Verification items for the finished model (mm, model axes). A direction names the side the tool comes from. Give positions to 0.01 mm unless a question says otherwise; leave off trailing zeros. Write each loop counter-clockwise with the first axis right and the second up, starting at its lowest first coordinate (ties: lowest second). Pieces come first, ordered by that corner, then holes. Notation, with made-up numbers: (-30, 24) - (8, 24) arc R19 ccw to (8, 45) - close; hole circle Ø3 at (6, -16.5). An arc over 180 degrees is marked (long way). Put each result on its own line as item: value.
from build123d import *

# Parameters (mm, degrees)
IZIM1_R                     = 1.5
IZIM1_R_2                   = 1.275
Y_KSEKLIK_EKSTR_ZYON1_DEPTH = 8
IZIM2_R                     = 4
KES_EKSTR_ZYON1_DEPTH       = 5
IZIM3_R                     = 3.5
KES_EKSTR_ZYON2_DEPTH       = 5
IZIM5_W                     = 11.833700998
IZIM5_H                     = 5.687133077
Y_KSEKLIK_EKSTR_ZYON2_DEPTH = 49
IZIM6_R                     = 1.5
KES_EKSTR_ZYON3_DEPTH       = 70
IZIM7_R                     = 7.94785764
KES_EKSTR_ZYON4_DEPTH       = 94.5
IZIM8_R                     = 2.303053837
IZIM8_R_2                   = 1.275
Y_KSEKLIK_EKSTR_ZYON3_DEPTH = 7
IZIM9_W                     = 9.184473095
IZIM9_H                     = 54.60219781
KES_EKSTR_ZYON5_DEPTH       = 49


with BuildPart() as part:
    # Çizim1 → Yükseklik-Ekstrüzyon1 (new body)
    with BuildSketch(Plane.XY):
        with BuildLine():
            Line((-26.942326891, 14.769848309), (-7.118223783, 14.769848309))
            ThreePointArc((-7.118223783, 14.769848309), (-3.582689877, 13.305382214), (-2.118223783, 9.769848309))
            Line((-2.118223783, 9.769848309), (-2.118223783, -8.006371062))
            ThreePointArc((-2.118223783, -8.006371062), (-3.582689877, -11.541904968), (-7.118223783, -13.006371062))
            Line((-7.118223783, -13.006371062), (-26.942326891, -13.006371062))
            ThreePointArc((-26.942326891, -13.006371062), (-30.477860797, -14.470837156), (-31.942326891, -18.006371062))
            Line((-31.942326891, -18.006371062), (-31.942326891, -21.470074229))
            ThreePointArc((-31.942326891, -21.470074229), (-31.6091093, -24.030019123), (-30.63166332, -26.419360282))
            Line((-30.63166332, -26.419360282), (-25.398075072, -35.607838889))
            ThreePointArc((-25.398075072, -35.607838889), (-21.734031643, -39.304154624), (-16.708738643, -40.658552836))
            Line((-16.708738643, -40.658552836), (16.824084861, -40.658552836))
            ThreePointArc((16.824084861, -40.658552836), (21.849377861, -39.304154624), (25.513421289, -35.607838889))
            Line((25.513421289, -35.607838889), (30.747009537, -26.419360282))
            ThreePointArc((30.747009537, -26.419360282), (31.724455518, -24.030019123), (32.057673109, -21.470074229))
            Line((32.057673109, -21.470074229), (32.057673109, -18.006371062))
            ThreePointArc((32.057673109, -18.006371062), (30.593207015, -14.470837156), (27.057673109, -13.006371062))
            Line((27.057673109, -13.006371062), (7.233570001, -13.006371062))
            ThreePointArc((7.233570001, -13.006371062), (3.698036095, -11.541904968), (2.233570001, -8.006371062))
            Line((2.233570001, -8.006371062), (2.233570001, 9.769848309))
            ThreePointArc((2.233570001, 9.769848309), (3.698036095, 13.305382214), (7.233570001, 14.769848309))
            Line((7.233570001, 14.769848309), (27.057673109, 14.769848309))
            ThreePointArc((27.057673109, 14.769848309), (30.593207015, 16.234314403), (32.057673109, 19.769848309))
            Line((32.057673109, 19.769848309), (32.057673109, 23.233551476))
            ThreePointArc((32.057673109, 23.233551476), (31.724455518, 25.793496369), (30.747009537, 28.182837528))
            Line((30.747009537, 28.182837528), (25.513421289, 37.371316135))
            ThreePointArc((25.513421289, 37.371316135), (21.849377861, 41.06763187), (16.824084861, 42.422030083))
            Line((16.824084861, 42.422030083), (-16.708738643, 42.422030083))
            ThreePointArc((-16.708738643, 42.422030083), (-21.734031643, 41.06763187), (-25.398075072, 37.371316135))
            Line((-25.398075072, 37.371316135), (-30.63166332, 28.182837528))
            ThreePointArc((-30.63166332, 28.182837528), (-31.6091093, 25.793496369), (-31.942326891, 23.233551476))
            Line((-31.942326891, 23.233551476), (-31.942326891, 19.769848309))
            ThreePointArc((-31.942326891, 19.769848309), (-30.477860797, 16.234314403), (-26.942326891, 14.769848309))
        make_face()
        with Locations((20.284256069, 32.422030083)):
            Circle(IZIM1_R, mode=Mode.SUBTRACT)
        with Locations((-20.168909852, 32.422030083)):
            Circle(IZIM1_R, mode=Mode.SUBTRACT)
        with Locations((-20.168909852, -30.658552836)):
            Circle(IZIM1_R, mode=Mode.SUBTRACT)
        with Locations((20.284256069, -30.658552836)):
            Circle(IZIM1_R, mode=Mode.SUBTRACT)
        with Locations((22.057673109, -21.118261377)):
            Circle(IZIM1_R_2, mode=Mode.SUBTRACT)
        with Locations((-21.942326891, -21.118261377)):
            Circle(IZIM1_R_2, mode=Mode.SUBTRACT)
        with Locations((22.057673109, 22.881738623)):
            Circle(IZIM1_R_2, mode=Mode.SUBTRACT)
        with Locations((-21.942326891, 22.881738623)):
            Circle(IZIM1_R_2, mode=Mode.SUBTRACT)
        with Locations((0.057673109, 32.422030083)):
            Circle(IZIM1_R, mode=Mode.SUBTRACT)
        with Locations(Location((0.057673109, -30.658552836, 0), (0, 0, 180))):
            Circle(IZIM1_R, mode=Mode.SUBTRACT)
    extrude(amount=Y_KSEKLIK_EKSTR_ZYON1_DEPTH)

    # Çizim2 → Kes-Ekstrüzyon1 (cut)
    with BuildSketch(Plane(origin=(0, 0, 0), x_dir=(-1, 0, 0), z_dir=(0, 0, -1))):
        with Locations((-22.057673109, 22.881738623)):
            Circle(IZIM2_R)
        with Locations((21.942326891, 22.881738623)):
            Circle(IZIM2_R)
        with Locations((-22.057673109, -21.118261377)):
            Circle(IZIM2_R)
        with Locations((21.942326891, -21.118261377)):
            Circle(IZIM2_R)
        with Locations((-0.057673109, 32.422030083)):
            Circle(IZIM2_R)
        with Locations((-0.057673109, -30.658552836)):
            Circle(IZIM2_R)
    extrude(amount=-KES_EKSTR_ZYON1_DEPTH, mode=Mode.SUBTRACT)

    # Çizim3 → Kes-Ekstrüzyon2 (cut)
    with BuildSketch(Plane.XY.offset(8)):
        with Locations((-20.168909852, 32.422030083)):
            Circle(IZIM3_R)
        with Locations((20.284256069, 32.422030083)):
            Circle(IZIM3_R)
        with Locations((20.284256069, -30.658552836)):
            Circle(IZIM3_R)
        with Locations((-20.168909852, -30.658552836)):
            Circle(IZIM3_R)
    extrude(amount=-KES_EKSTR_ZYON2_DEPTH, mode=Mode.SUBTRACT)

    # Çizim5 → Yükseklik-Ekstrüzyon2 (add)
    with BuildSketch(Plane.XY.offset(8)):
        with Locations((0.057673109, 32.422030083)):
            Rectangle(IZIM5_W, IZIM5_H)
        with Locations((0.057673109, -30.658552837)):
            Rectangle(IZIM5_W, IZIM5_H)
    extrude(amount=Y_KSEKLIK_EKSTR_ZYON2_DEPTH)

    # Çizim6 → Kes-Ekstrüzyon3 (cut)
    with BuildSketch(Plane(origin=(0, 0, 8), x_dir=(-1, 0, 0), z_dir=(0, 0, -1))):
        with Locations((-0.057673109, -30.658552836)):
            Circle(IZIM6_R)
        with Locations((-0.057673109, 32.422030083)):
            Circle(IZIM6_R)
    extrude(amount=-KES_EKSTR_ZYON3_DEPTH, mode=Mode.SUBTRACT)

    # Çizim7 → Kes-Ekstrüzyon4 (cut, symmetric)
    with BuildSketch(Plane.XY.offset(8)):
        with Locations((30.593207015, 16.234314403)):
            Circle(IZIM7_R)
        with Locations((-30.477860797, 16.234314403)):
            Circle(IZIM7_R)
        with Locations((30.593207015, -14.470837156)):
            Circle(IZIM7_R)
        with Locations((-30.477860797, -14.470837156)):
            Circle(IZIM7_R)
    extrude(amount=KES_EKSTR_ZYON4_DEPTH, both=True, mode=Mode.SUBTRACT)

    # Çizim8 → Yükseklik-Ekstrüzyon3 (add)
    # profile 1 of 4: a face of its own
    with BuildSketch(Plane.XY.offset(8)):
        with Locations((-21.942326891, 22.881738623)):
            Circle(IZIM8_R)
        with Locations(Location((-21.942326891, 22.881738623, 0), (0, 0, 180))):
            Circle(IZIM8_R_2, mode=Mode.SUBTRACT)
    # profile 2 of 4: a face of its own
    with BuildSketch(Plane.XY.offset(8)):
        with Locations((22.057673109, 22.881738623)):
            Circle(IZIM8_R)
        with Locations(Location((22.057673109, 22.881738623, 0), (0, 0, 180))):
            Circle(IZIM8_R_2, mode=Mode.SUBTRACT)
    # profile 3 of 4: a face of its own
    with BuildSketch(Plane.XY.offset(8)):
        with Locations((-21.942326891, -21.118261377)):
            Circle(IZIM8_R)
        with Locations(Location((-21.942326891, -21.118261377, 0), (0, 0, 180))):
            Circle(IZIM8_R_2, mode=Mode.SUBTRACT)
    # profile 4 of 4: a face of its own
    with BuildSketch(Plane.XY.offset(8)):
        with Locations((22.057673109, -21.118261377)):
            Circle(IZIM8_R)
        with Locations(Location((22.057673109, -21.118261377, 0), (0, 0, 180))):
            Circle(IZIM8_R_2, mode=Mode.SUBTRACT)
    extrude(amount=Y_KSEKLIK_EKSTR_ZYON3_DEPTH)

    # Çizim9 → Kes-Ekstrüzyon5 (cut, symmetric)
    with BuildSketch(Plane(origin=(2.233570001, 0, 0), x_dir=(0, 0, -1), z_dir=(1, 0, 0))):
        with Locations((0.592236548, 0.881738623)):
            Rectangle(IZIM9_W, IZIM9_H)
    extrude(amount=KES_EKSTR_ZYON5_DEPTH, both=True, mode=Mode.SUBTRACT)


solid = part.part
Q1. Section check B-B, the plane x = -11.5. Record the cut outline in (y, z), plus the area to 3 significant figures.
Answers follow:
outline: (-40.66, 0) - (-26.42, 0) - (-26.42, 4) - (-13.01, 4) - (-13.01, 8) - (-40.66, 8) - close; (14.77, 4) - (28.18, 4) - (28.18, 0) - (42.42, 0) - (42.42, 8) - (14.77, 8) - close
area: 335 mm2
Q2. Section check A-A, the plane z = 17. Record the cut outline in (x, y).
Answers follow:
outline: (-5.86, -33.5) - (5.97, -33.5) - (5.97, -27.81) - (-5.86, -27.81) - close; (-5.86, 29.58) - (5.97, 29.58) - (5.97, 35.27) - (-5.86, 35.27) - close; hole circle Ø3 at (0.06, -30.66); hole circle Ø3 at (0.06, 32.42)
Q3. Section check C-C, the plane z = 11. Give the number of separate pieces and of enclosed holes in the cut face, plus the area to 3 significant figures.
Answers follow:
separate pieces: 6
enclosed holes: 6
area: 167 mm2
Q4. Scan lines: line 1 along X through (y, z) = (23, 11); line 2 along Y through (x, z) = (-1.5, 48); line 3 along Y through (x, z) = (-0.5, 15). Record each from-to range of solid material in increasing order.
Answers follow:
line 1: x = -24.24 to -23.21, -20.67 to -19.64, 19.76 to 20.79, 23.33 to 24.36
line 2: y = -33.5 to -27.81, 29.58 to 35.27
line 3: y = -33.5 to -32.05, -29.27 to -27.81, 29.58 to 31.03, 33.81 to 35.27
Q5. Set-up check for faces 1 (the face through (22, 32, 3)), 2 (the face through (0.1, -32.4, 5)), 3 (the face through (0, 35.266, 32)), 4 (the face through (21.79, -39.34, 3.94)), 5 (the face through (-3.54, -11.5, 5.97)): record each of +Z, -Z, +X, -X, +Y, -Y from which the full face is reachable in a straight line by a thin tool's end or side.
Answers follow:
face 1: +Z
face 2: -Z
face 3: +Z, +X, -X, +Y
face 4: +Z, -Z, +X, -Y
face 5: +Z, -Z, -X
Q6. Release check for a two-part mould opening along X. For faces 6 (the face through (0, 42.422, 4)), 7 (the face through (28.17, 32.71, 3.94)), 8 (the face through (25.04, 21.92, 6.03)), 9 (the face through (3.232, -33.092, 2.465)) record: released by +X, released by -X, zero draft, split by the parting line, or undercut.
Answers follow:
face 6: zero draft
face 7: released by +X
face 8: undercut
face 9: undercut
Q7. Section check D-D, the plane y = 5.5. Record the cut outline in (x, z), plus the area to 3 significant figures.
Answers follow:
outline: (-2.12, 4) - (2.23, 4) - (2.23, 8) - (-2.12, 8) - close
area: 17.4 mm2
Q8. Go/stop test with flat-tipped pins: pin 1 Ø5.5 at (x, y) = (19, -32) entering from +Z; pin 2 Ø3 at (y, z) = (-1.5, 6.5) entering from +X; pin 3 Ø6 at (y, z) = (30, 31.5) entering from -X; pin 4 Ø2.5 at (x, y) = (-20.17, -30.66) entering from -Z. Record where each tip stops, or that it passes through.
Answers follow:
pin 1: stops at z = 8
pin 2: stops at x = 2.23
pin 3: stops at x = -5.86
pin 4: passes through
